Here's how the part is built. I have some questions about the finished solid (model axes, mm). A direction names the side the tool comes from. Coordinates: 2 decimals unless noted, no trailing zeros. Write each loop counter-clockwise with the first axis right and the second up, starting at its lowest first coordinate (ties: lowest second). Pieces come first, ordered by that corner, then holes. Notation, with made-up numbers: (-1.75, 79) - (26.25, 79) arc R25 cw to (26.25, 111) - close; hole circle Ø2 at (-25, 66). An arc over 180 degrees is marked (long way). Answer in a Markdown table with one row per item. Add a question column.
Item 1: If I drill on probe 1 along Z at (x, y) = (-42, -10); probe 2 along Z at (x, y) = (-75.5, -85); probe 3 along Y at (x, z) = (-80, 66), over which ranges is the centre line in solid material (lowest first)? Write a range as from..to.
Item 2: Imagine slicing it at C-C (z = 9). Please give me the cut outline in (x, y).
Item 3: I'm going to push flat-ended pins straight in: pin 1 (25 mm diameter, centred on y = -16.5, z = 42, fed in from +X); pin 2 (10 mm diameter, centred on x = -30, y = -55, fed in from +Z); pin 3 (13 mm diameter, centred on x = -56.5, z = 9.5, fed in from -Y). Where does each tip first touch, or does it pass through?
Item 4: We'd pull the mould along X, two halves only. Please class faces 4 (the face through (-13.784, -16, 42)), 5 (the face through (-93.235, -40, 23)), 6 (the face through (-54, -30.988, 45)), 7 (the face through (-52, -16, 47.907)): +X half, -X half, draft (parallel to the pull), parting line (faces both ways), or undercut.
Item 5: Imagine slicing it at B-B (y = -10). Please give me the cut outline in (x, z).
Item 6: Which directions (+Z, -Z, +X, -X, +Y, -Y) give clear straight access to the entire face, cutting with the end or side of a thin tool? Please do faces 1 (the face through (-58, -76.454, 13)), 2 (the face through (-65.902, -16, 61)), 3 (the face through (-18.227, -15.711, 67.081)).
Item 7: Imagine slicing it at A-A (z = 49.5). Please give me the cut outline in (x, y), plus the area to 3 significant figures.
Item 8: Imagine slicing it at D-D (x = -69). Please give me the cut outline in (y, z).
from build123d import *

# Parameters (mm, degrees)
F0_W      = 101.6
F0_H      = 101.6
F1_DEPTH  = 75.438
F2_W      = 28.0288234353
F2_H      = 9.1542927548
F3_DEPTH  = 25.4
F4_W      = 101.6
F4_H      = 49.6587024246
F5_DEPTH  = 70.612
F6_W      = 27.8729833663
F6_H      = 25.5314931273
F7_DEPTH  = 25.146
F9_DEPTH  = 68.072
F10_DEPTH = 25.4
F12_DEPTH = 60.96
F13_W     = 27.6737101376
F13_H     = 27.5311653678
F14_DEPTH = 72.136
F15_DEPTH = 13.716
F16_DEPTH = 13.462
F18_DEPTH = 43.434


with BuildPart() as f1:
    # F0 (on Top) → F1 (new body)
    with BuildSketch(Plane.XY):
        with Locations((-50.8, -50.8)):
            Rectangle(F0_W, F0_H)
    extrude(amount=F1_DEPTH)

    # F2 (on face) → F3 (cut)
    with BuildSketch(Plane.XZ.offset(101.6)):
        with Locations((-57.5784109533, -4.5771463774)):
            Rectangle(F2_W, F2_H)
    extrude(amount=-F3_DEPTH, mode=Mode.SUBTRACT)

    # F4 (on face) → F5 (cut)
    with BuildSketch(Plane.XZ.offset(101.6)):
        with Locations((-50.8, 50.6086487877)):
            Rectangle(F4_W, F4_H)
    extrude(amount=-F5_DEPTH, mode=Mode.SUBTRACT)

    # F6 (on face) → F7 (cut)
    with BuildSketch(Plane.XZ.offset(101.6)):
        with Locations((-57.6563309878, 13.0135510117)):
            Rectangle(F6_W, F6_H)
    extrude(amount=-F7_DEPTH, mode=Mode.SUBTRACT)

    # F8 (on face) → F9 (cut)
    with BuildSketch(Plane.XZ.offset(30.988)):
        Polygon((-93.2351276278, 58.4865286946), (-78.3963426948, 75.438), (-101.6, 75.438), (-101.6, 25.7792975754), (-93.2351276278, 25.7792975754), align=None)
    extrude(amount=-F9_DEPTH, mode=Mode.SUBTRACT)

    # F10 (cut): a face of the model
    f10_faces = [f1.faces().sort_by_distance(p)[0] for p in [
        (-57.6563309878, -89.027, 0.247804448),
    ]]
    extrude(f10_faces, amount=-F10_DEPTH, mode=Mode.SUBTRACT)

    # F11 (on face) → F12 (cut)
    with BuildSketch(Plane.XZ.offset(30.988)):
        Polygon((0, 75.438), (-22.546928376, 75.438), (-13.7835862115, 58.4865286946), (-13.7835862115, 25.7792975754), (0, 25.7792975754), align=None)
    extrude(amount=-F12_DEPTH, mode=Mode.SUBTRACT)

    # F13 (on face) → F14 (cut)
    with BuildSketch(Plane.XZ.offset(30.988)):
        with Locations((-52.0655419677, 61.6724173161)):
            Rectangle(F13_W, F13_H)
    extrude(amount=-F14_DEPTH, mode=Mode.SUBTRACT)

    # F15 (add): a face of the model
    f15_faces = [f1.faces().sort_by_distance(p)[0] for p in [
        (0, -50.8, 12.8896487877),
    ]]
    extrude(f15_faces, amount=-F15_DEPTH)

    # F16 (cut): a face of the model
    f16_faces = [f1.faces().sort_by_distance(p)[0] for p in [
        (0, -50.8, 12.8896487877),
    ]]
    extrude(f16_faces, amount=-F16_DEPTH, mode=Mode.SUBTRACT)

    # F17 (on face) → F18 (cut)
    with BuildSketch(Plane.XY.offset(25.7792975754)):
        Polygon((-93.2351276278, -101.6), (-93.2351276278, -30.988), (-93.2351276278, 0), (-101.6, 0), (-101.6, -101.6), align=None)
    extrude(amount=-F18_DEPTH, mode=Mode.SUBTRACT)


solid = f1.part
Here are the results:
| question | item | result |
|---|---|---|
| 1 | probe 1 | z = 0..47.91 |
| 1 | probe 2 | z = 0..25.78 |
| 1 | probe 3 | y = -30.99..0 |
| 2 | outline | (-93.24, -101.6) - (-71.59, -101.6) - (-71.59, -76.45) - (-43.72, -76.45) - (-43.72, -101.6) - (-13.46, -101.6) - (-13.46, 0) - (-93.24, 0) - close |
| 3 | pin 1 | stops at x = -13.78 |
| 3 | pin 2 | stops at z = 25.78 |
| 3 | pin 3 | stops at y = -76.45 |
| 4 | face 4 | +X half |
| 4 | face 5 | -X half |
| 4 | face 6 | draft |
| 4 | face 7 | undercut |
| 5 | outline | (-93.24, 0) - (-13.46, 0) - (-13.46, 25.78) - (-13.78, 25.78) - (-13.78, 58.49) - (-22.55, 75.44) - (-38.23, 75.44) - (-38.23, 47.91) - (-65.9, 47.91) - (-65.9, 75.44) - (-78.4, 75.44) - (-93.24, 58.49) - close |
| 6 | face 1 | +Z, -Z, -Y |
| 6 | face 2 | +Z, +Y, -Y |
| 6 | face 3 | +Z, +X, +Y, -Y |
| 7 | outline | (-93.24, -30.99) - (-65.9, -30.99) - (-65.9, 0) - (-93.24, 0) - close; (-38.23, -30.99) - (-13.78, -30.99) - (-13.78, 0) - (-38.23, 0) - close |
| 7 | area | 1,600 mm2 |
| 8 | outline | (-76.45, 0) - (0, 0) - (0, 75.44) - (-30.99, 75.44) - (-30.99, 25.78) - (-76.45, 25.78) - close |
